from build123d import *

# Parameters (mm, degrees)
F0_W     = 38.1
F0_H     = 38.1
F1_DEPTH = 38.1
F3_DEPTH = 38.1
F2_W     = 12.7
F2_H     = 6.35
F4_DEPTH = 38.1


with BuildPart() as f1:
    # F0 (on Top) → F1 (new body)
    with BuildSketch(Plane.XY):
        with Locations((19.05, 19.05)):
            Rectangle(F0_W, F0_H)
    extrude(amount=F1_DEPTH)

    # F2 (on face) → F3 (cut)
    with BuildSketch(Plane.YZ.offset(38.1)):
        Polygon((0, 38.1), (0, 0), (12.681324, 38.1), align=None)
    extrude(amount=-F3_DEPTH, mode=Mode.SUBTRACT)

    # F2 (on face) → F4 (cut)
    with BuildSketch(Plane.YZ.offset(38.1)):
        Polygon((25.4, 38.1), (38.1, 0), (38.1, 38.1), align=None)
        with Locations((19.05, 3.175)):
            Rectangle(F2_W, F2_H)
        Polygon((0, 38.1), (0, 0), (12.681324, 38.1), align=None)
    extrude(amount=-F4_DEPTH, mode=Mode.SUBTRACT)


solid = f1.part
Work out the finished part from the listing and answer in its coordinate system (mm). A direction names the side the tool comes from. Coordinates: 2 decimals unless noted, no trailing zeros. Order: outer loops, then holes, each group sorted by start corner. A loop starts at its lowest first (then second) coordinate and runs counter-clockwise, first axis right, second up. Notation, with made-up numbers: (-33.5, 1) - (-14.5, 1) arc R20 ccw to (-14.5, 18) - close; hole circle Ø3 at (34, 42.25). An arc over 180 degrees is marked (long way). Put each result on its own line as item: value. Start each with the question number.
1) For a pull along Y with two mould halves and no side action, classify faces 1 (the flat face through (19.32, 6.25, 18.78)), 2 (the flat face through (38.1, 19, 19)), 3 (the flat face through (19, 19, 6.35)), 4 (the flat face through (19.32, 31.66, 19.32)) as released by +Y, released by -Y, zero draft, split by the parting line, or undercut.
2) Find the intervals of material crossed by line 1 (Z direction, x = 20, y = 13); line 2 (Y direction, x = 15, z = 5); line 3 (Y direction, x = 36.5, z = 21), in increasing order. Write a range as from..to.
3) For faces 5 (the flat face through (19, 12.7, 3)), 6 (the flat face through (19, 19, 38.1)), determine the directions among +Z, -Z, +X, -X, +Y, -Y from which every point of the face is accessible in a straight line to the end or side of a thin tool.
4) Flat-ended cylindrical pins translate along their axes: pin 1 (1.5 mm diameter, centred on x = 28, y = 16, fed in from -Z); pin 2 (8 mm diameter, centred on x = 14, z = 31.5, fed in from -Y); pin 3 (12 mm diameter, centred on x = 31.5, z = 16.5, fed in from +Y). Find the tip coordinate at first contact, or state that the pin passes through.
5) Find section C-C (z = 13). Give the vertices of the cut face in (x, y).
6) Find section A-A (x = 21.5). Give the vertices of the cut face in (y, z), plus the area to 3 significant figures.
7) Find section B-B (y = 35). Give the vertices of the cut face in (x, z), plus the area to 3 significant figures.
Results list:
1. face 1: released by -Y
1. face 2: zero draft
1. face 3: undercut
1. face 4: released by +Y
2. line 1: z = 6.35..38.1
2. line 2: y = 1.66..12.7, 25.4..36.43
2. line 3: y = 6.99..31.1
3. face 5: -Z, +X, -X
3. face 6: +Z, +X, -X, +Y, -Y
4. pin 1: stops at z = 6.35
4. pin 2: stops at y = 9.15
4. pin 3: stops at y = 34.6
5. outline: (0, 4.33) - (38.1, 4.33) - (38.1, 33.77) - (0, 33.77) - close
6. outline: (0, 0) - (12.7, 0) - (12.7, 6.35) - (25.4, 6.35) - (25.4, 0) - (38.1, 0) - (25.4, 38.1) - (12.68, 38.1) - close
6. area: 887 mm^2
7. outline: (0, 0) - (38.1, 0) - (38.1, 9.3) - (0, 9.3) - close
7. area: 354 mm^2
